Here's the drawing with two shaded views (mm, measured from the low corner). I have some questions. A direction names the side the tool comes from. Give positions to 0.01 mm unless a question says otherwise; leave off trailing zeros. Order: outer loops, then holes, each group sorted by start corner. A loop starts at its lowest first (then second) coordinate and runs counter-clockwise, first axis right, second up. Notation, with made-up numbers: (78.5, 55.25) - (99.5, 55.25) arc R17 cw to (99.5, 85.25) - close; hole circle Ø9 at (7, 48). An arc over 180 degrees is marked (long way). Use one line per item in the form item = value. Start each with the question number.
1) Suppose I cut it at C-C, the plane z = 1. Write out the boundary of the cut face in (x, y) (3 decimals), and give its area (3 significant figures).
2) Which directions (+Z, -Z, +X, -X, +Y, -Y) give clear straight access to the entire face, cutting with the end or side of a thin tool? Please do the marked faces 1 and 2.
3) Please list where these lines run through material, in increasing order: probe 1 along Z at (x, y) = (2.87, 1); probe 2 along Y at (x, z) = (5, 3.5); probe 3 along Y at (x, z) = (25, 2.25).
4) For pin 1 (5 mm diameter, centred on x = 18.5, z = 2, fed in from +Y); pin 2 (4 mm diameter, centred on x = 10.5, z = 6, fed in from -Y); pin 3 (3 mm diameter, centred on x = 21, z = 3, fed in from -Y); pin 4 (0.6 mm diameter, centred on x = 20.5, y = 3.5, fed in from +Z), each with a flat end and sliding along its axis, tell me the tip position at first contact or that it passes through.
5) Suppose I cut it at B-B, the plane z = 5.27. Write out the boundary of the cut face in (x, y) (3 decimals), and give its area (3 significant figures).
6) Suppose I cut it at A-A, the plane x = 2.87. Write out the boundary of the cut face in (y, z), and give its area (3 significant figures).
7) Suppose I cut it at D-D, the plane x = 21.5. Write out the boundary of the cut face in (y, z), and give its area (3 significant figures).
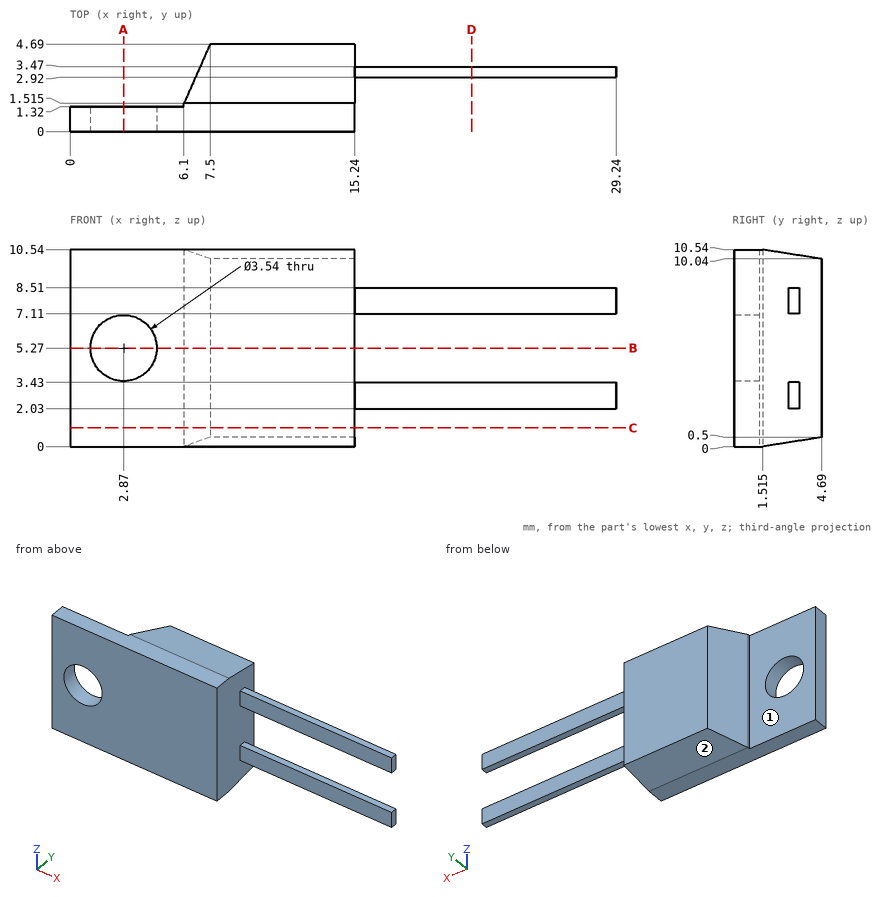
Result sheet:
q1.outline = (0, 0) - (15.24, 0) - (15.24, 4.69) - (7.5, 4.69) - (6.1, 1.515) - (6.1, 1.32) - (0, 1.32) - close
q1.area = 48.7 mm²
q2.face_1 = +Z, -Z, -X, +Y
q2.face_2 = -Z, +X, -X, +Y
q3.probe_1 = 0 to 3.5, 7.04 to 10.54
q3.probe_2 = 0 to 1.32
q3.probe_3 = 2.92 to 3.47
q4.pin_1 = 3.47
q4.pin_2 = 0
q4.pin_3 = 2.92
q4.pin_4 = 8.51
q5.outline = (0, 0) - (1.1, 0) - (1.1, 1.32) - (0, 1.32) - close; (4.64, 0) - (15.24, 0) - (15.24, 4.69) - (7.5, 4.69) - (6.1, 1.515) - (6.1, 1.32) - (4.64, 1.32) - close
q5.area = 44.0 mm²
q6.outline = (0, 0) - (1.32, 0) - (1.32, 3.5) - (0, 3.5) - close; (0, 7.04) - (1.32, 7.04) - (1.32, 10.54) - (0, 10.54) - close
q6.area = 9.24 mm²
q7.outline = (2.92, 2.03) - (3.47, 2.03) - (3.47, 3.43) - (2.92, 3.43) - close; (2.92, 7.11) - (3.47, 7.11) - (3.47, 8.51) - (2.92, 8.51) - close
q7.area = 1.54 mm²
